For this review, take the finished solid that the model builds, in its own axes (mm). Face numbers are marked on the shaded views. Coordinates: 2 decimals unless noted, no trailing zeros. Order: outer loops, then holes, each group sorted by start corner. A loop starts at its lowest first (then second) coordinate and runs counter-clockwise, first axis right, second up. Notation, with made-up numbers: (8.5, 52) -> (58.5, 52) arc R13 ccw to (58.5, 77) -> close; hole circle Ø1 at (52, -36.75). An arc over 180 degrees is marked (long way). Return JSON: item names as keys, results as strings. Group by question number.
Item 1: Take a section at B-B (y = -7.5). Write out the cut boundary in (x, z).
Item 2: For line 1 along X through (y, z) = (-2.5, -25.4); line 2 along Z through (x, y) = (25.4, -7); line 3 along Z through (x, y) = (21.5, -11.75) (3 decimals), list the stretches that pass through material, from the lowest coordinate up.
Item 3: Draft analysis for pull direction Z (two halves, no side actions). For the marked faces 1, 2 and 3, state which applies: +Z half, -Z half, draft (parallel to the pull), parting line (faces both ways), or undercut.
Item 4: Insertion check: pin 1 (4 mm diameter, centred on x = 33.5, z = -32.5, fed in from -Y). The pin has a flat end and moves straight along its axis. Give the tip position at first contact, or say it passes through.
Item 5: Take a section at A-A (z = -25.4). Write out the cut boundary in (x, y) (3 decimals).
Item 6: Take a section at C-C (x = 25.4). Write out the cut boundary in (y, z) (3 decimals).
Item 7: Take a section at D-D (x = 47). Write out the cut boundary in (y, z) (3 decimals).
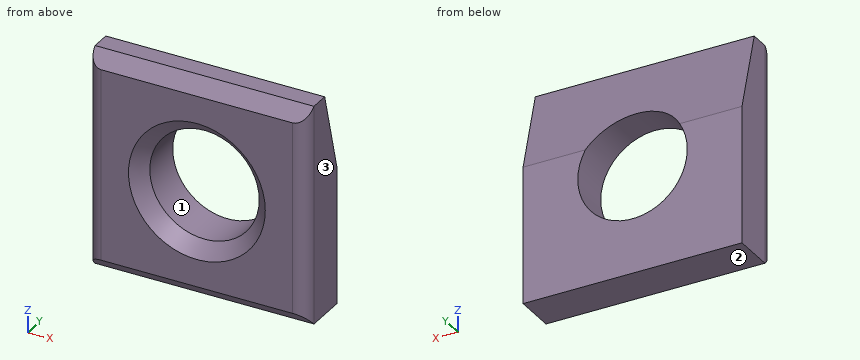
```python
from build123d import *

# Parameters (mm, degrees)
F0_W        = 50.8
F0_H        = 50.8
F1_DEPTH    = 12.7
F2_R        = 12.7
F3_DEPTH    = 25.4
F4_R        = 3.175
F5_T1_DEPTH = 60.7801869736
F6_T1_DEPTH = 149.2615438243


# Not quite as in the source:
# - a fillet or chamfer that OpenCascade refuses, or shapes differently, is made with other operations: its cross-section is extruded or revolved along the edge and cut away or added


with BuildPart() as f1:
    # F0 (on Front) → F1 (new body)
    with BuildSketch(Plane.XZ):
        with Locations((25.4, -25.4)):
            Rectangle(F0_W, F0_H)
    extrude(amount=F1_DEPTH)

    # F2 (on face) → F3 (cut)
    with BuildSketch(Plane.XZ.offset(12.7)):
        with Locations((25.4, -25.4)):
            Circle(F2_R)
    extrude(amount=-F3_DEPTH, mode=Mode.SUBTRACT)

    # F4
    f4_edges = [f1.edges().sort_by_distance(p)[0] for p in [
        (0, -12.7, -25.4),
        (50.8, -12.7, -25.4),
    ]]
    fillet(f4_edges, radius=F4_R)

    # F5: chamfer of 3.175 on 3 edges, made by hand

    # F5_s2 → F5_t1 (cut)
    with BuildSketch(Plane.YZ.offset(-4.9900934868)):
        Polygon((-9.525, 0), (-12.7, -3.175), (-12.7, 0), align=None)
        Polygon((-12.7, -47.625), (-9.525, -50.8), (-12.7, -50.8), align=None)
    extrude(amount=F5_T1_DEPTH, mode=Mode.SUBTRACT)

    # F5_s3 → F5_t4 (revolve, cut)
    with BuildSketch(Plane.XY.offset(-25.4)):
        Polygon((41.275, -12.7), (38.1, -9.525), (38.1, -12.7), align=None)
    revolve(axis=Axis((25.4, -12.7, -25.4), (0, -1, 0)), mode=Mode.SUBTRACT)

    # F6: chamfer of 5.08 x 18.9588181024 on 1 edges, made by hand

    # F6_s2 → F6_t1 (cut)
    with BuildSketch(Plane.YZ.offset(-49.2307719121)):
        Polygon((-5.08, 0), (0, -18.9588181024), (0, 0), align=None)
    extrude(amount=F6_T1_DEPTH, mode=Mode.SUBTRACT)


solid = f1.part
```
Findings below:
{
 "1": {"outline": "(0, -50.8) -> (50.8, -50.8) -> (50.8, 0) -> (0, 0) -> close; hole circle Ø25.4 at (25.4, -25.4)"},
 "2": {"line 1": "x = 0 to 12.7, 38.1 to 50.8", "line 2": "z = -50.8 to -38.1, -12.7 to 0", "line 3": "z = -48.575 to -39.806, -10.994 to -2.225"},
 "3": {"face 1": "undercut", "face 2": "-Z half", "face 3": "draft"},
 "4": {"pin 1": "stops at y = -9.6"},
 "5": {"outline": "(0, -9.525) arc R3.175 ccw to (3.175, -12.7) -> (9.525, -12.7) -> (12.7, -9.525) -> (12.7, 0) -> (0, 0) -> close; (38.1, -9.525) -> (41.275, -12.7) -> (47.625, -12.7) arc R3.175 ccw to (50.8, -9.525) -> (50.8, 0) -> (38.1, 0) -> close"},
 "6": {"outline": "(-12.7, -47.625) -> (-9.525, -50.8) -> (0, -50.8) -> (0, -38.1) -> (-9.525, -38.1) -> (-12.7, -41.275) -> close; (-12.7, -9.525) -> (-9.525, -12.7) -> (-1.677, -12.7) -> (-5.08, 0) -> (-9.525, 0) -> (-12.7, -3.175) -> close"},
 "7": {"outline": "(-12.7, -47.625) -> (-9.525, -50.8) -> (0, -50.8) -> (0, -18.959) -> (-5.08, 0) -> (-9.525, 0) -> (-12.7, -3.175) -> close"}
}
